```python
from build123d import *

# Parameters (mm, degrees)
BOSS_EXTRUDE1_DEPTH = 3


with BuildPart() as part:
    # Sketch1 → Boss-Extrude1 (new body)
    with BuildSketch(Plane(origin=(0, 0, 0), x_dir=(1, 0, 0), z_dir=(0, 1, 0))):
        with BuildLine():
            Line((0, -8.5), (0, 0))
            ThreePointArc((0, 0), (-1.982516962, -0.146362799), (-3.922046259, -0.582277556))
            ThreePointArc((-3.922046259, -0.582277556), (-10.844298606, -5.459403769), (-13.5, -13.5))
            Line((-13.5, -13.5), (-11.5, -13.5))
            ThreePointArc((-11.5, -13.5), (-10, -12), (-8.5, -13.5))
            Line((-8.5, -13.5), (-5, -13.5))
            ThreePointArc((-5, -13.5), (-3.535533906, -9.964466094), (0, -8.5))
        make_face()
        with BuildLine():
            ThreePointArc((0, -18.5), (-3.535533906, -17.035533906), (-5, -13.5))
            Line((-5, -13.5), (-8.5, -13.5))
            ThreePointArc((-8.5, -13.5), (-10, -15), (-11.5, -13.5))
            Line((-11.5, -13.5), (-13.5, -13.5))
            ThreePointArc((-13.5, -13.5), (-10.844298606, -21.540596231), (-3.922046259, -26.417722444))
            ThreePointArc((-3.922046259, -26.417722444), (-1.982516962, -26.853637201), (0, -27))
            Line((0, -27), (0, -18.5))
        make_face()
        with BuildLine():
            ThreePointArc((-13.5, -13.5), (-10.844298606, -5.459403769), (-3.922046259, -0.582277556))
            Line((-3.922046259, -0.582277556), (-30, -8.5))
            Line((-30, -8.5), (-30, -13.5))
            Line((-30, -13.5), (-25.5, -13.5))
            ThreePointArc((-25.5, -13.5), (-24, -12), (-22.5, -13.5))
            Line((-22.5, -13.5), (-19.5, -13.5))
            ThreePointArc((-19.5, -13.5), (-18, -12), (-16.5, -13.5))
            Line((-16.5, -13.5), (-13.5, -13.5))
        make_face()
        with BuildLine():
            ThreePointArc((-3.922046259, -26.417722444), (-10.844298606, -21.540596231), (-13.5, -13.5))
            Line((-13.5, -13.5), (-16.5, -13.5))
            ThreePointArc((-16.5, -13.5), (-18, -15), (-19.5, -13.5))
            Line((-19.5, -13.5), (-22.5, -13.5))
            ThreePointArc((-22.5, -13.5), (-24, -15), (-25.5, -13.5))
            Line((-25.5, -13.5), (-30, -13.5))
            Line((-30, -13.5), (-30, -18.5))
            Line((-30, -18.5), (-3.922046259, -26.417722444))
        make_face()
        with BuildLine():
            ThreePointArc((3.922046259, -0.582277556), (1.982516962, -0.146362799), (0, 0))
            Line((0, 0), (0, -8.5))
            ThreePointArc((0, -8.5), (3.535533906, -9.964466094), (5, -13.5))
            Line((5, -13.5), (8.5, -13.5))
            ThreePointArc((8.5, -13.5), (10, -12), (11.5, -13.5))
            Line((11.5, -13.5), (13.5, -13.5))
            ThreePointArc((13.5, -13.5), (10.844298606, -5.459403769), (3.922046259, -0.582277556))
        make_face()
        with BuildLine():
            Line((8.5, -13.5), (5, -13.5))
            ThreePointArc((5, -13.5), (3.535533906, -17.035533906), (0, -18.5))
            Line((0, -18.5), (0, -27))
            ThreePointArc((0, -27), (1.982516962, -26.853637201), (3.922046259, -26.417722444))
            ThreePointArc((3.922046259, -26.417722444), (10.844298606, -21.540596231), (13.5, -13.5))
            Line((13.5, -13.5), (11.5, -13.5))
            ThreePointArc((11.5, -13.5), (10, -15), (8.5, -13.5))
        make_face()
        with BuildLine():
            Line((16.5, -13.5), (13.5, -13.5))
            ThreePointArc((13.5, -13.5), (10.844298606, -21.540596231), (3.922046259, -26.417722444))
            Line((3.922046259, -26.417722444), (30, -18.5))
            Line((30, -18.5), (30, -13.5))
            Line((30, -13.5), (25.5, -13.5))
            ThreePointArc((25.5, -13.5), (24, -15), (22.5, -13.5))
            Line((22.5, -13.5), (19.5, -13.5))
            ThreePointArc((19.5, -13.5), (18, -15), (16.5, -13.5))
        make_face()
        with BuildLine():
            Line((30, -8.5), (3.922046259, -0.582277556))
            ThreePointArc((3.922046259, -0.582277556), (10.844298606, -5.459403769), (13.5, -13.5))
            Line((13.5, -13.5), (16.5, -13.5))
            ThreePointArc((16.5, -13.5), (18, -12), (19.5, -13.5))
            Line((19.5, -13.5), (22.5, -13.5))
            ThreePointArc((22.5, -13.5), (24, -12), (25.5, -13.5))
            Line((25.5, -13.5), (30, -13.5))
            Line((30, -13.5), (30, -8.5))
        make_face()
    extrude(amount=BOSS_EXTRUDE1_DEPTH)


solid = part.part
```
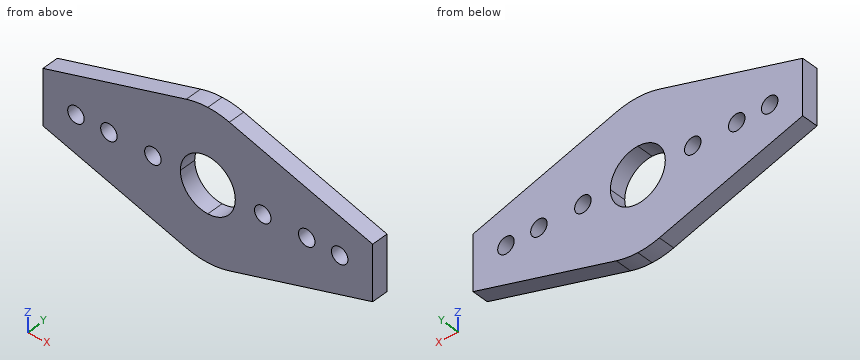
Can you work these out from the model? Positions are in its coordinate system, mm. Give positions to 0.01 mm unless a question says otherwise; leave off trailing zeros. Order: outer loops, then holes, each group sorted by start corner. A loop starts at its lowest first (then second) coordinate and runs counter-clockwise, first axis right, second up. Notation, with made-up numbers: M 17.25,71 L 64.25,71 A25 cw 64.25,92 Z; hole C -19.75,-37.75 d3. An arc over 180 degrees is marked long. One line per item, written item: value.
1) I want a section at C-C, the plane z = 17.75. List the corners of the cut face in (x, y) for me, plus the area to 3 significant figures.
Answer sheet:
outline: M -30,0 L -2.63,0 L -2.63,3 L -30,3 Z; M 2.63,0 L 30,0 L 30,3 L 2.63,3 Z
area: 164 mm^2
2) Please list where these lines run through material, in increasing order: line 1 along Z through (x, y) = (18, 2.3); line 2 along X through (y, z) = (2.6, 10.5); line 3 along X through (y, z) = (1.6, 9.5).
Answer sheet:
line 1: z = 4.86 to 12, 15 to 22.14
line 2: x = -30 to -4, 4 to 30
line 3: x = -30 to -3, 3 to 30
3) I want a section at B-B, the plane x = -10. List the corners of the cut face in (y, z) for me.
Answer sheet:
outline: M 0,2.43 L 3,2.43 L 3,12 L 0,12 Z; M 0,15 L 3,15 L 3,24.57 L 0,24.57 Z
4) I want a section at A-A, the plane y = 1.9. List the corners of the cut face in (x, z) for me.
Answer sheet:
outline: M -30,8.5 L -3.92,0.58 A13.5 ccw 3.92,0.58 L 30,8.5 L 30,18.5 L 3.92,26.42 A13.5 ccw -3.92,26.42 L -30,18.5 Z; hole C -24,13.5 d3; hole C -18,13.5 d3; hole C -10,13.5 d3; hole C 0,13.5 d10; hole C 10,13.5 d3; hole C 18,13.5 d3; hole C 24,13.5 d3
5) For P1, Ø1.8, axis at x = -18, z = 13.5, coming from the -Y side; P2, Ø1, axis at x = -5.5, y = 0.5, coming from the -Z side, each with a flat end and sliding along its axis, tell me the tip position at first contact or that it passes through.
Answer sheet:
P1: passes through
P2: stops at z = 0.91
